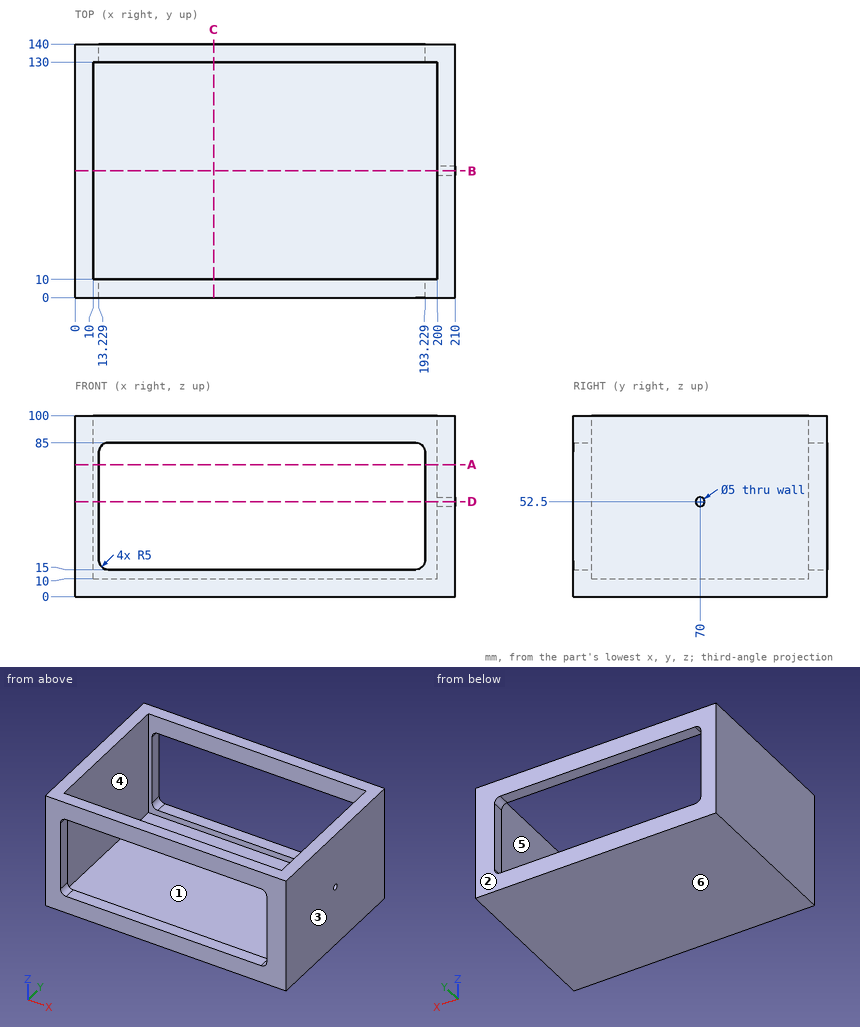
Check sheet for the drawn part. Datum: minimum x, y, z corner. Units: mm. A direction names the side the tool comes from. Round coordinates to 2 decimals unless told otherwise and drop trailing zeros. Order: outer loops, then holes, each group sorted by start corner. A loop starts at its lowest first (then second) coordinate and runs counter-clockwise, first axis right, second up.
1. Access from +Z, -Z, +X, -X, +Y, -Y to the whole of each face (thin tool, end or side, straight path). Record for the marked faces 5 and 6.
Final values:
face 5: +Z
face 6: -Z, +X, -X, +Y, -Y
2. Thickness scan on L1, parallel to Z at x = 206.75, y = 70; L2, parallel to Y at x = 206, z = 52.5; L3, parallel to X at y = 58.5, z = 38.5. Record the ranges inside material, lowest first.
Final values:
L1: z = 0 to 50, 55 to 100
L2: y = 0 to 67.5, 72.5 to 140
L3: x = 0 to 10, 200 to 210
3. Section check B-B on y = 70. Record the cut outline in (x, z).
Final values:
outline: (0, 0) - (210, 0) - (210, 50) - (200, 50) - (200, 10) - (10, 10) - (10, 100) - (0, 100) - close; (200, 55) - (210, 55) - (210, 100) - (200, 100) - close
4. Section check D-D on z = 52.5. Record the cut outline in (x, y), then the cut area to 3 significant figures.
Final values:
outline: (0, 0) - (13.23, 0) - (13.23, 10) - (10, 10) - (10, 130) - (13.23, 130) - (13.23, 140) - (0, 140) - close; (193.23, 0) - (210, 0) - (210, 67.5) - (200, 67.5) - (200, 10) - (193.23, 10) - close; (193.23, 130) - (200, 130) - (200, 72.5) - (210, 72.5) - (210, 140) - (193.23, 140) - close
area: 2,950 mm2
5. Section check C-C on x = 76.5. Record the cut outline in (y, z), then the cut area to 3 significant figures.
Final values:
outline: (0, 0) - (140, 0) - (140, 15) - (130, 15) - (130, 10) - (10, 10) - (10, 15) - (0, 15) - close; (0, 85) - (10, 85) - (10, 100) - (0, 100) - close; (130, 85) - (140, 85) - (140, 100) - (130, 100) - close
area: 1,800 mm2
6. Release check for a two-part mould opening along X. For the marked faces 1, 2, 3 and 4 record: +X half, -X half, draft (parallel to the pull), parting line (faces both ways), or undercut.
Final values:
face 1: undercut
face 2: draft
face 3: +X half
face 4: undercut
7. Go/stop test with flat-tipped pins: P1, Ø5, axis at x = 88, y = 111.5, coming from the +Z side; P2, Ø5, axis at y = 137, z = 56.5, coming from the -X side. Record where each tip stops, or that it passes through.
Final values:
P1: stops at z = 10
P2: stops at x = 0
8. Section check A-A on z = 73. Record the cut outline in (x, y), then the cut area to 3 significant figures.
Final values:
outline: (0, 0) - (13.23, 0) - (13.23, 10) - (10, 10) - (10, 130) - (13.23, 130) - (13.23, 140) - (0, 140) - close; (193.23, 0) - (210, 0) - (210, 140) - (193.23, 140) - (193.23, 130) - (200, 130) - (200, 10) - (193.23, 10) - close
area: 3,000 mm2
